For this review, take the finished solid that the model builds, in its own axes (mm). Give positions to 0.01 mm unless a question says otherwise; leave off trailing zeros. Order: outer loops, then holes, each group sorted by start corner. A loop starts at its lowest first (then second) coordinate and runs counter-clockwise, first axis right, second up. Notation, with made-up numbers: M -20,-28 L 36,-28 A18 ccw 36,-3 Z; hole C 17.25,-22.5 d11. An arc over 180 degrees is marked long. Use CSV: the item, a comma, the result in double quotes. Start each with the question number.
(1) Consider section D-D (z = -2.2). Give the number of separate pieces and of enclosed holes in the cut face, and give its area (3 significant figures).
(2) Consider section C-C (x = 67.45). Write out the cut boundary in (y, z), and give its area (3 significant figures).
(3) Wall thickness on L1, parallel to X at y = 66, z = -1.8; L2, parallel to X at y = 17, z = -2.25; L3, parallel to Y at x = 67.45, z = -2.05: over which ranges is each line inside the solid? List them lowest first. Write a range as from..to.
(4) Consider section A-A (y = 33.5). Write out the cut boundary in (x, z), and give its area (3 significant figures).
(5) Consider section B-B (x = 118.4). Write out the cut boundary in (y, z).
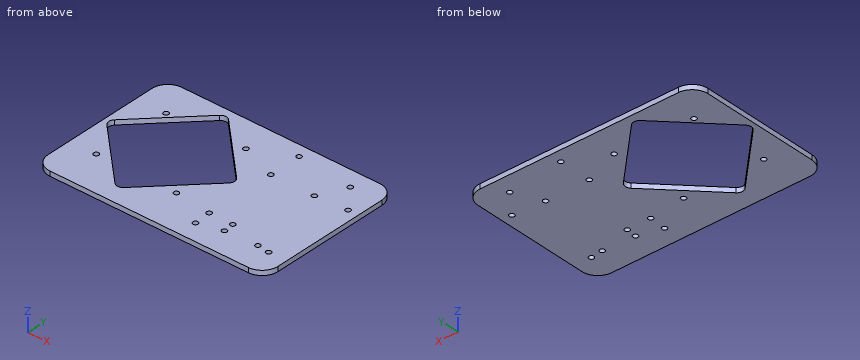
```python
from build123d import *

# Parameters (mm, degrees)
ESQUISSE1_R               = 1.6
T_LE_DE_BASE_PLI_E1_DEPTH = 3


# Sheet-metal steps are written as plain solids
with BuildPart() as part:
    # Esquisse1 → Tôle de base pliée1 (new body)
    with BuildSketch(Plane.XY):
        with BuildLine():
            Line((10, 0), (135, 0))
            ThreePointArc((135, 0), (142.071067812, 2.928932188), (145, 10))
            Line((145, 10), (145, 85))
            ThreePointArc((145, 85), (142.071067812, 92.071067812), (135, 95))
            Line((135, 95), (10, 95))
            ThreePointArc((10, 95), (2.928932188, 92.071067812), (0, 85))
            Line((0, 85), (0, 10))
            ThreePointArc((0, 10), (2.928932188, 2.928932188), (10, 0))
        make_face()
        with Locations((90.9, 87.2)):
            Circle(ESQUISSE1_R, mode=Mode.SUBTRACT)
        with Locations((126.368886423, 83.535840528)):
            Circle(ESQUISSE1_R, mode=Mode.SUBTRACT)
        with Locations((138.5, 68.05)):
            Circle(ESQUISSE1_R, mode=Mode.SUBTRACT)
        with Locations((118.4, 66.74856953)):
            Circle(ESQUISSE1_R, mode=Mode.SUBTRACT)
        with Locations((90.9, 66.74856953)):
            Circle(ESQUISSE1_R, mode=Mode.SUBTRACT)
        with Locations((126.1, 17.1)):
            Circle(ESQUISSE1_R, mode=Mode.SUBTRACT)
        with Locations((133.7, 16.15)):
            Circle(ESQUISSE1_R, mode=Mode.SUBTRACT)
        with Locations((105.3, 22.8)):
            Circle(ESQUISSE1_R, mode=Mode.SUBTRACT)
        with Locations((90.4, 22.8)):
            Circle(ESQUISSE1_R, mode=Mode.SUBTRACT)
        with Locations((91.1, 12.1)):
            Circle(ESQUISSE1_R, mode=Mode.SUBTRACT)
        with Locations((105.9, 16.1)):
            Circle(ESQUISSE1_R, mode=Mode.SUBTRACT)
        with Locations((67.45, 25.4)):
            Circle(ESQUISSE1_R, mode=Mode.SUBTRACT)
        with Locations((19, 73.4)):
            Circle(ESQUISSE1_R, mode=Mode.SUBTRACT)
        with Locations((16.9, 25.4)):
            Circle(ESQUISSE1_R, mode=Mode.SUBTRACT)
        with Locations((67.45, 75.6)):
            Circle(ESQUISSE1_R, mode=Mode.SUBTRACT)
        with BuildLine():
            Line((44.882149159, 88.890256032), (80.590443676, 53.891431727))
            ThreePointArc((80.590443676, 53.891431727), (81.790336387, 51.074901862), (80.647201293, 48.234862221))
            Line((80.647201293, 48.234862221), (45.648376988, 12.526567705))
            ThreePointArc((45.648376988, 12.526567705), (42.831847123, 11.326674993), (39.991807483, 12.469810088))
            Line((39.991807483, 12.469810088), (4.283512966, 47.468634392))
            ThreePointArc((4.283512966, 47.468634392), (3.083620254, 50.285164258), (4.226755349, 53.125203898))
            Line((4.226755349, 53.125203898), (39.225579653, 88.833498415))
            ThreePointArc((39.225579653, 88.833498415), (42.042109519, 90.033391126), (44.882149159, 88.890256032))
        make_face(mode=Mode.SUBTRACT)
    extrude(amount=-T_LE_DE_BASE_PLI_E1_DEPTH)


solid = part.part
```
Check result:
1,separate pieces,"1"
1,enclosed holes,"16"
1,area,"10,200 mm^2"
2,outline,"M 0,-3 L 23.8,-3 L 23.8,0 L 0,0 Z; M 27,-3 L 34.77,-3 L 34.77,0 L 27,0 Z; M 66.77,-3 L 74,-3 L 74,0 L 66.77,0 Z; M 77.2,-3 L 95,-3 L 95,0 L 77.2,0 Z"
2,area,"170 mm^2"
3,L1,"x = 0..16.85, 68.24..89.49, 92.31..116.99, 119.81..145"
3,L2,"x = 0..35.37, 50.03..104.58, 107.22..124.5, 127.7..132.34, 135.06..145"
3,L3,"y = 0..23.8, 27..34.77, 66.77..74, 77.2..95"
4,outline,"M 0,-3 L 18.54,-3 L 18.54,0 L 0,0 Z; M 66.21,-3 L 145,-3 L 145,0 L 66.21,0 Z"
4,area,"292 mm^2"
5,outline,"M 0,-3 L 65.15,-3 L 65.15,0 L 0,0 Z; M 68.35,-3 L 95,-3 L 95,0 L 68.35,0 Z"
